Job drawing, mm, ordinate dimensions from the low corner. One solid piece. A direction names the side the tool comes from. Give positions to 0.01 mm unless a question says otherwise; leave off trailing zeros. Order: outer loops, then holes, each group sorted by start corner. A loop starts at its lowest first (then second) coordinate and runs counter-clockwise, first axis right, second up.
Item 1: Flat gauge pins, fed straight in: P1, Ø8, axis at y = 10, z = 33, coming from the -X side; P2, Ø3, axis at x = 26.57, z = 10.5, coming from the +Y side; P3, Ø12, axis at y = 15.5, z = 26, coming from the -X side. Where does each tip first touch, or does it go through?
Item 2: Band-saw the part on B-B on x = 12. Give the cut face in (y, z), plus the area to 3 significant figures.
Item 3: Band-saw the part on A-A on z = 10.5. Give the cut face in (x, y).
Item 4: Band-saw the part on C-C on x = 5.57. Give the cut face in (y, z) (1 decimal).
Item 5: Which spindle directions (+Z, -Z, +X, -X, +Y, -Y) get a long thin tool onto all of the face, cutting with end or side? Do the marked faces 4 and 5. Say none if no direction does.
Item 6: Band-saw the part on D-D on z = 16. Give the cut face in (x, y).
Item 7: Wall check: L1, parallel to Z at x = 20.5, y = 7.75; L2, parallel to Y at x = 29.6, z = 6 (1 decimal); L3, parallel to X at y = 0.75, z = 10.5. Give the ranges that are in metal, low to high.
Item 8: Two-plate mould, pull along Z, no slides. Class the marked faces 1, 2 and 3: released by +Z, released by -Z, zero draft, split by the parting line, or undercut.
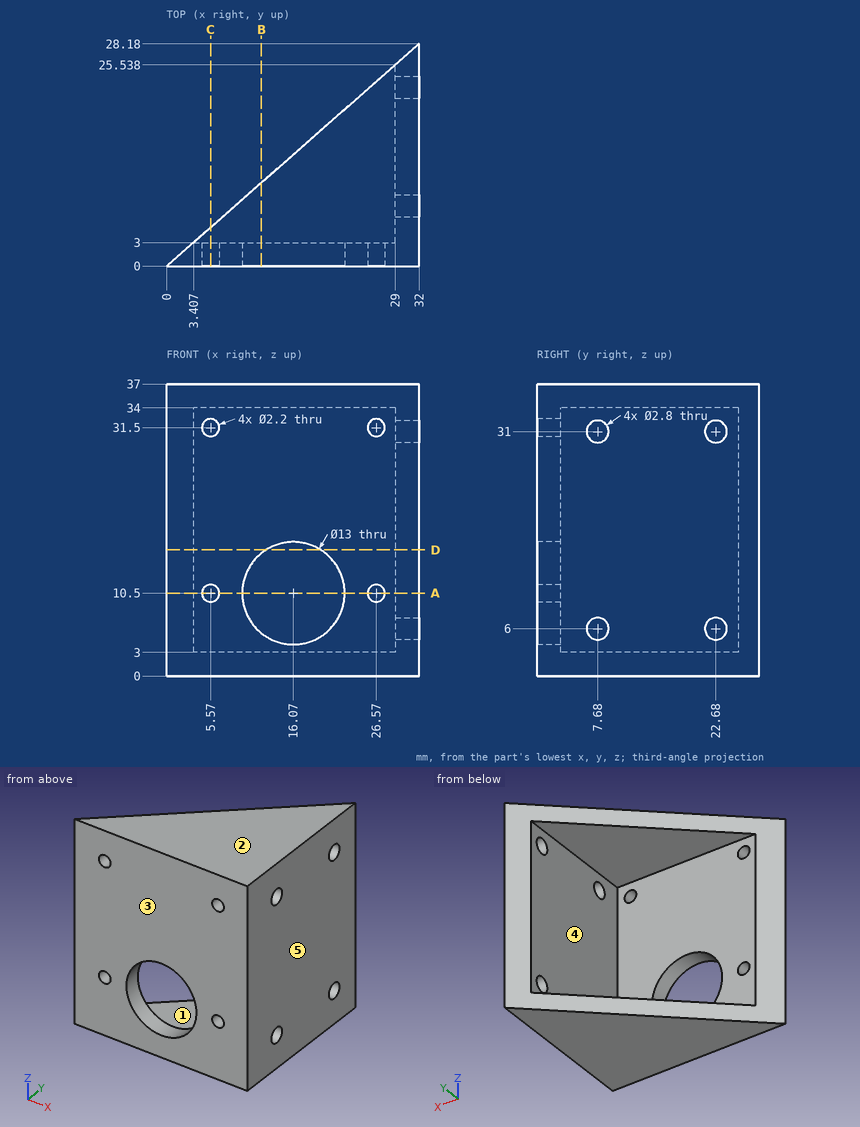
The answers:
1. P1: stops at x = 6.96
1. P2: stops at y = 3
1. P3: stops at x = 29
2. outline: (0, 0) - (10.57, 0) - (10.57, 3) - (3, 3) - (3, 5.43) - (0, 5.43) - close; (0, 15.57) - (3, 15.57) - (3, 34) - (10.57, 34) - (10.57, 37) - (0, 37) - close
2. area: 126 mm2
3. outline: (0, 0) - (4.47, 0) - (4.47, 3) - (3.41, 3) - close; (6.67, 0) - (9.57, 0) - (9.57, 3) - (6.67, 3) - close; (22.57, 0) - (25.47, 0) - (25.47, 3) - (22.57, 3) - close; (27.67, 0) - (32, 0) - (32, 28.18) - (29, 25.54) - (29, 3) - (27.67, 3) - close
4. outline: (0, 0) - (4.9, 0) - (4.9, 3) - (3, 3) - (3, 9.4) - (0, 9.4) - close; (0, 11.6) - (3, 11.6) - (3, 30.4) - (0, 30.4) - close; (0, 32.6) - (3, 32.6) - (3, 34) - (4.9, 34) - (4.9, 37) - (0, 37) - close
5. face 4: -X, +Y
5. face 5: +Z, -Z, +X, +Y, -Y
6. outline: (0, 0) - (12.61, 0) - (12.61, 3) - (3.41, 3) - close; (19.53, 0) - (32, 0) - (32, 28.18) - (29, 25.54) - (29, 3) - (19.53, 3) - close
7. L1: z = 0 to 3, 34 to 37
7. L2: y = 0 to 6.3, 9.1 to 21.3, 24.1 to 26.1
7. L3: x = 0.85 to 4.47, 6.67 to 9.57, 22.57 to 25.47, 27.67 to 32
8. face 1: undercut
8. face 2: released by +Z
8. face 3: zero draft
